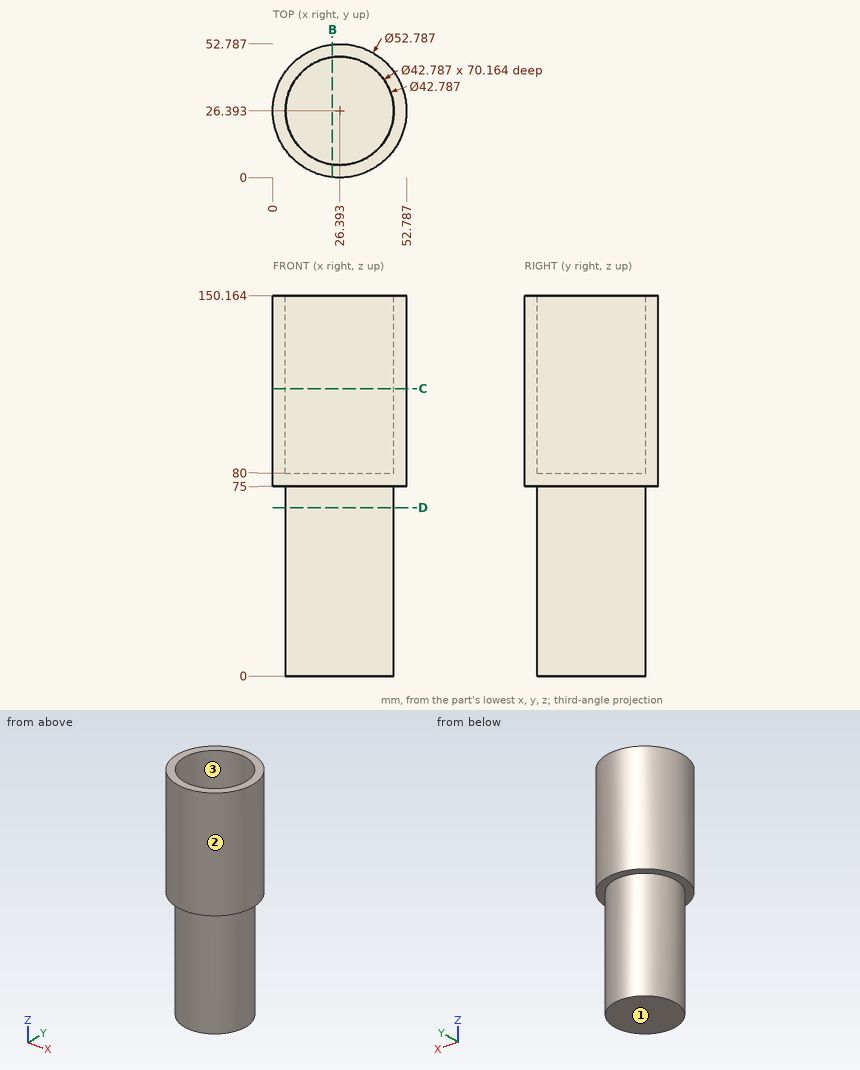
Answer from the drawing. Dimensions are ordinates in mm from the lowest x, y and z of the part. Coordinates: 2 decimals unless noted, no trailing zeros. Write each loop counter-clockwise with the first axis right and the second up, starting at its lowest first coordinate (ties: lowest second). Pieces come first, ordered by that corner, then holes. Notation, with made-up numbers: (-29.5, -34) - (29.5, -34) arc R18 ccw to (29.5, -11) - close; hole circle Ø6 at (-35, 25.5). An arc over 180 degrees is marked (long way). Return JSON: item names as keys, results as strings. Group by question number.
Q1. The part is cut by section B-B on x = 23.5. Write down the section's boundary in (y, z), and give its area (3 significant figures).
Q2. The part is cut by section D-D on z = 66.5. Write down the section's boundary in (x, y), and give its area (3 significant figures).
Q3. Find the intervals of material crossed by line 1 along Y through (x, z) = (26, 139.5); line 2 along X through (y, z) = (27.5, 123.5); line 3 along Z through (x, y) = (22, 16), in increasing order. Write a range as [from, to].
Q4. Flat-ended cylindrical pins translate along their axes: pin 1 Ø5 at (y, z) = (30, 42) entering from -X; pin 2 Ø4 at (y, z) = (23.5, 70.5) entering from +X; pin 3 Ø4 at (x, z) = (13.5, 43.5) entering from +Y (1 decimal). Find the tip coordinate at first contact, or state that the pin passes through.
Q5. The part is cut by section C-C on z = 113.5. Write down the section's boundary in (x, y).
Q6. For a pull along X with two mould halves and no side action, classify the marked faces 1, 2 and 3 as +X half, -X half, draft (parallel to the pull), parting line (faces both ways), or undercut.
Evaluation:
{
 "1": {"outline": "(0.16, 75) - (5.2, 75) - (5.2, 0) - (47.59, 0) - (47.59, 75) - (52.63, 75) - (52.63, 150.16) - (47.59, 150.16) - (47.59, 80) - (5.2, 80) - (5.2, 150.16) - (0.16, 150.16) - close", "area": "4,150 mm2"},
 "2": {"outline": "circle Ø42.79 at (26.39, 26.39)", "area": "1,440 mm2"},
 "3": {"line 1": "y = [0, 5], [47.78, 52.78]", "line 2": "x = [0.02, 5.03], [47.76, 52.76]", "line 3": "z = [0, 80]"},
 "4": {"pin 1": "stops at x = 5.03", "pin 2": "stops at x = 47.77", "pin 3": "stops at y = 44.8"},
 "5": {"outline": "circle Ø52.79 at (26.39, 26.39); hole circle Ø42.79 at (26.39, 26.39)"},
 "6": {"face 1": "draft", "face 2": "parting line", "face 3": "undercut"}
}
